```python
from build123d import *

# Parameters (mm, degrees)
SKETCH012_W      = 320
SKETCH012_H      = 12
EXTRUDE001_DEPTH = 4
SKETCH007_W      = 12
SKETCH007_H      = 40
SKETCH007_W_2    = 40
SKETCH007_H_2    = 12
EXTRUDE_DEPTH    = 12


with BuildPart() as innertemplatealignmentslot:
    # Sketch012 → Extrude001 (new body)
    with BuildSketch(Plane.XY):
        with Locations((0, -6)):
            Rectangle(SKETCH012_W, SKETCH012_H)
    extrude(amount=EXTRUDE001_DEPTH)


with BuildPart() as innertemplatealignmentslot_1:
    # Extrude001 placement: moved
    add(innertemplatealignmentslot.part.moved(Location((0, 0, 8))))


with BuildPart() as innertemplate:
    # Sketch007 → Extrude (new body)
    with BuildSketch(Plane.XY):
        with BuildLine():
            ThreePointArc((160, 0), (0, 160), (-160, 0))
            Line((-160, 0), (-160, -100))
            Line((-160, -100), (160, -100))
            Line((160, -100), (160, 0))
        make_face()
        Polygon((-140, -72.5), (-95, -72.5), (-95, -27.5), (-140, -27.5), (-140, -50), align=None, mode=Mode.SUBTRACT)
        Polygon((-136.272177, 32.091959), (-94.697598, 14.871205), (-77.476843, 56.445784), (-119.051422, 73.666538), (-127.6618, 52.879249), align=None, mode=Mode.SUBTRACT)
        Polygon((-32.091959, 136.272177), (-14.871205, 94.697598), (-56.445784, 77.476843), (-73.666538, 119.051422), (-52.879249, 127.6618), align=None, mode=Mode.SUBTRACT)
        Polygon((73.666538, 119.051422), (56.445784, 77.476843), (14.871205, 94.697598), (32.091959, 136.272177), (52.879249, 127.6618), align=None, mode=Mode.SUBTRACT)
        Polygon((136.272177, 32.091959), (94.697598, 14.871205), (77.476843, 56.445784), (119.051422, 73.666538), (127.6618, 52.879249), align=None, mode=Mode.SUBTRACT)
        Polygon((94.999107, -27.5), (139.999107, -27.5), (139.999107, -50), (139.999107, -72.5), (94.999107, -72.5), align=None, mode=Mode.SUBTRACT)
        Polygon((66.390873, -27.5), (66.390873, 27.5), (27.5, 66.390873), (-27.5, 66.390873), (-66.390873, 27.5), (-66.390873, -27.5), align=None, mode=Mode.SUBTRACT)
        Polygon((-94.661353, 103.146635), (-66.377082, 74.862363), (-74.862363, 66.377082), (-103.146635, 94.661353), (-98.903994, 98.903994), align=None, mode=Mode.SUBTRACT)
        with Locations((0, 119.871369)):
            Rectangle(SKETCH007_W, SKETCH007_H, mode=Mode.SUBTRACT)
        Polygon((103.146635, 94.661353), (74.862363, 66.377082), (66.377082, 74.862363), (94.661353, 103.146635), (98.903994, 98.903994), align=None, mode=Mode.SUBTRACT)
        with Locations((-120, -6)):
            Rectangle(SKETCH007_W_2, SKETCH007_H_2, mode=Mode.SUBTRACT)
        with Locations((119.999107, -6.5)):
            Rectangle(SKETCH007_W_2, SKETCH007_H_2, mode=Mode.SUBTRACT)
        with Locations((0, -73.5)):
            Rectangle(SKETCH007_W_2, SKETCH007_H_2, mode=Mode.SUBTRACT)
    extrude(amount=EXTRUDE_DEPTH)

    # Cut: cut InnerTemplateAlignmentSlot
    add(innertemplatealignmentslot_1.part, mode=Mode.SUBTRACT)


with BuildPart() as innertemplate_1:
    # Cut placement: moved
    add(innertemplate.part.moved(Location((0, 0, 6))))


solid = innertemplate_1.part
```
Geometry: final body of the model. Coordinates: model frame, mm. A direction names the side the tool comes from. Give positions to 0.01 mm unless a question says otherwise; leave off trailing zeros. Loops run counter-clockwise (first coordinate to the right, second up) from the corner with the lowest first, then second, coordinate; pieces in that order, holes last. Notation, with made-up numbers: (14.25, 16.25) -> (31.25, 16.25) arc R21 ccw to (31.25, 52.25) -> close; hole circle Ø1 at (53, 67.5). An arc over 180 degrees is marked (long way). Use one line per item in the form item = value.
Item 1: Access query for faces 3 (the face through (-1, -27.5, 12)), 4 (the face through (-150, -6, 14)), 5 (the face through (-160, -49, 12)). Directions: +Z, -Z, +X, -X, +Y, -Y. A direction counts if a zero-diameter tool reaches every point of the face in a straight line with its end or side. Return the directions, or none.
A:
face_3 = +Z, -Z
face_4 = +Z, +X, -X
face_5 = +Z, -Z, -X, +Y, -Y
Item 2: Pin query (flat end, axial travel): P1, Ø6, axis at y = 117.5, z = 12, coming from the -X side; P2, Ø2, axis at x = 79.5, z = 16.5, coming from the +Y side; P3, Ø3.5, axis at x = -81.5, y = -9, coming from the +Z side. Return the tip coordinate at first contact, or that it passes through.
A:
P1 = -111.76
P2 = 139.42
P3 = 14
Item 3: Line query: probe 1 along X at (y, z) = (49, 13.75); probe 2 along X at (y, z) = (-22, 12.25); probe 3 along Y at (x, z) = (-62.5, 14.75). Output: solid intervals per line, ascending.
A:
probe_1 = -152.31 to -129.27, -80.56 to -44.89, 44.89 to 80.56, 129.27 to 152.31
probe_2 = -160 to -66.39, 66.39 to 160
probe_3 = -100 to -27.5, 31.39 to 92.09, 123.68 to 147.29
Item 4: Draft query along Y for faces 1 (the face through (160, -51, 12)), 2 (the face through (-140, -6, 10)). Return one class per face: pulls with the +Y half, pulls with the -Y half, needs draft (parallel to the pull), parting line crosses it, or undercut.
A:
face_1 = needs draft
face_2 = undercut
Item 5: Section query A-A on x = 0. Output: boundary loops of the cut face in (y, z), and give its area (3 significant figures).
A:
outline = (-100, 6) -> (-79.5, 6) -> (-79.5, 18) -> (-100, 18) -> close; (-67.5, 6) -> (-27.5, 6) -> (-27.5, 18) -> (-67.5, 18) -> close; (66.39, 6) -> (99.87, 6) -> (99.87, 18) -> (66.39, 18) -> close; (139.87, 6) -> (160, 6) -> (160, 18) -> (139.87, 18) -> close
area = 1,370 mm^2
Item 6: Section query C-C on y = 114. Output: boundary loops of the cut face in (x, z).
A:
outline = (-112.27, 6) -> (-71.57, 6) -> (-71.57, 18) -> (-112.27, 18) -> close; (-22.87, 6) -> (-6, 6) -> (-6, 18) -> (-22.87, 18) -> close; (6, 6) -> (22.87, 6) -> (22.87, 18) -> (6, 18) -> close; (71.57, 6) -> (112.27, 6) -> (112.27, 18) -> (71.57, 18) -> close
Item 7: Section query B-B on y = -52. Output: boundary loops of the cut face in (x, z), and give its area (3 significant figures).
A:
outline = (-160, 6) -> (-140, 6) -> (-140, 18) -> (-160, 18) -> close; (-95, 6) -> (95, 6) -> (95, 18) -> (-95, 18) -> close; (140, 6) -> (160, 6) -> (160, 18) -> (140, 18) -> close
area = 2,760 mm^2
Item 8: Section query D-D on z = 10. Give the number of separate pieces and of enclosed holes in the cut face, and give its area (3 significant figures).
A:
separate_pieces = 1
enclosed_holes = 13
area = 46,200 mm^2
